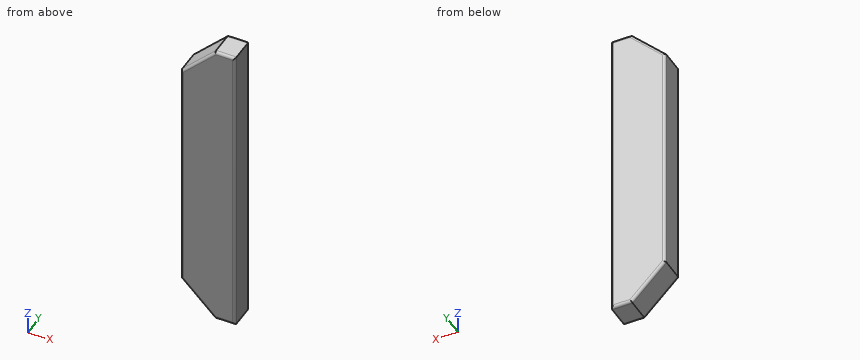
from build123d import *

# Parameters (mm, degrees)
SKETCH2_W           = 101.6
SKETCH2_H           = 50.8
BOSS_EXTRUDE1_DEPTH = 575.4
CUT_EXTRUDE1_DEPTH  = 51.8
FILLET1_R           = 5.08


with BuildPart() as part:
    # Sketch2 → Boss-Extrude1 (new body)
    with BuildSketch(Plane(origin=(0, 0, 287.7), x_dir=(-1, 0, 0), z_dir=(0, 0, -1))):
        with Locations((-2663.5, 12.7)):
            Rectangle(SKETCH2_W, SKETCH2_H)
    extrude(amount=BOSS_EXTRUDE1_DEPTH)

    # Sketch5 → Cut-Extrude1 (cut, through all)
    with BuildSketch(Plane(origin=(0, 38.1, 0), x_dir=(1, 0, 0), z_dir=(0, 1, 0))):
        Polygon((2612.7, -287.7), (2676.2, -287.7), (2612.7, -224.2), align=None)
        Polygon((2676.2, 287.7), (2612.7, 224.2), (2612.7, 287.7), align=None)
    extrude(amount=-CUT_EXTRUDE1_DEPTH, mode=Mode.SUBTRACT)

    # Fillet1
    fillet1_edges = [part.edges().sort_by_distance(p)[0] for p in [
        (2714.3, 38.1, 0),
        (2695.25, 38.1, -287.7),
        (2714.3, -12.7, 0),
        (2695.25, -12.7, -287.7),
        (2612.7, -12.7, 0),
        (2612.7, 38.1, 0),
        (2695.25, 38.1, 287.7),
        (2644.45, -12.7, -255.95),
        (2644.45, 38.1, -255.95),
        (2644.45, -12.7, 255.95),
        (2644.45, 38.1, 255.95),
        (2695.25, -12.7, 287.7),
    ]]
    fillet(fillet1_edges, radius=FILLET1_R)


solid = part.part
Work out the finished part from the listing and answer in its coordinate system (mm). Round coordinates to 2 decimals unless told otherwise and drop trailing zeros. Order: outer loops, then holes, each group sorted by start corner. A loop starts at its lowest first (then second) coordinate and runs counter-clockwise, first axis right, second up. Notation, with made-up numbers: M 38,24 L 95,24 A24 cw 95,63 Z; hole C 87,66 d4. An arc over 180 degrees is marked long. One line per item, written item: value.
Q1. Straight lines are drawn through the part: line 1 (X direction, y = 34, z = 200.5); line 2 (X direction, y = -8, z = 119.5); line 3 (Z direction, x = 2663, y = 28). For each, find the intervals that lie inside material, in ascending order.
Derived:
line 1: 2612.8 to 2714.2
line 2: 2612.71 to 2714.29
line 3: -274.5 to 274.5
Q2. A flat-ended cylindrical pin translates along its axis: pin 1 (8 mm diameter, centred on x = 2627.5, y = 28, fed in from +Z). Find the tip coordinate at first contact, or state that the pin passes through.
Derived:
pin 1: z = 243
Q3. Find section A-A on y = 15.5. Write down the section's boundary in (x, z), then the cut area to 3 significant figures.
Derived:
outline: M 2612.7,-224.2 L 2676.2,-287.7 L 2714.3,-287.7 L 2714.3,287.7 L 2676.2,287.7 L 2612.7,224.2 Z
area: 54,400 mm²
